Work out the finished part from the listing and answer in its coordinate system (mm). Round coordinates to 2 decimals unless told otherwise and drop trailing zeros. Order: outer loops, then holes, each group sorted by start corner. A loop starts at its lowest first (then second) coordinate and runs counter-clockwise, first axis right, second up. Notation, with made-up numbers: (86.25, 69) - (97.25, 69) arc R18 ccw to (97.25, 91) - close; hole circle Ø5 at (33.5, 63.5). An arc over 180 degrees is marked (long way). Put each result on its own line as item: value.
```python
from build123d import *

# Parameters (mm, degrees)
F0_W     = 31.75
F0_H     = 12.7
F1_DEPTH = 66.675
F2_R     = 1.5875
F3_DEPTH = 25.4
F4_W     = 9.525
F4_H     = 3.175
F5_DEPTH = 3.175


with BuildPart() as f1:
    # F0 (on Front) → F1 (new body)
    with BuildSketch(Plane.XZ):
        with Locations((-96.787434, -12.355283)):
            Rectangle(F0_W, F0_H)
    extrude(amount=F1_DEPTH)

    # F2 (on face) → F3 (cut)
    with BuildSketch(Plane.XZ.offset(66.675)):
        with Locations((-88.027969, -9.819109)):
            Circle(F2_R)
    extrude(amount=-F3_DEPTH, mode=Mode.SUBTRACT)

    # F4 (on face) → F5 (cut)
    with BuildSketch(Plane.XY.offset(-6.005283)):
        with Locations((-100.361299, -63.160878)):
            Rectangle(F4_W, F4_H)
    extrude(amount=-F5_DEPTH, mode=Mode.SUBTRACT)


solid = f1.part
```
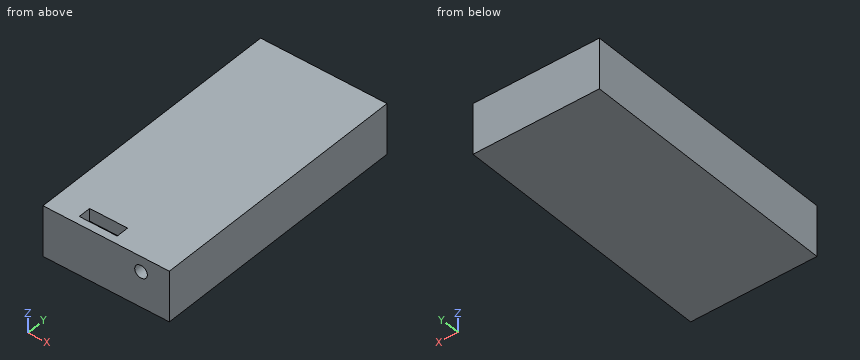
1) A cutting plane is placed at A-A on y = -53.5. Write down the section's boundary in (x, z) (1 decimal), then the cut area to 3 significant figures.
Findings below:
outline: (-112.7, -18.7) - (-80.9, -18.7) - (-80.9, -6) - (-112.7, -6) - close; hole circle Ø3.2 at (-88, -9.8)
area: 395 mm2
2) Straight lines are drawn through the part: L1, parallel to Y at x = -102.5, z = -8.25 (3 decimals); L2, parallel to Y at x = -88, z = -8.75 (3 decimals). For each, find the intervals that lie inside material, in ascending order. Write a range as from..to.
Findings below:
L1: y = -66.675..-64.748, -61.573..0
L2: y = -41.275..0
3) Given pin 1 Ø1.9 at (x, z) = (-88.03, -9.82) entering from -Y (3 decimals); pin 2 Ø1 at (x, y) = (-101, -63.5) entering from +Z, each flat-ended and moving along its own axis, determine where each tip first touches the part or whether it passes through.
Findings below:
pin 1: stops at y = -41.275
pin 2: stops at z = -9.18
